Drawing for the job (mm, zero at the part's lowest x, y, z). A direction names the side the tool comes from. Round coordinates to 2 decimals unless told otherwise and drop trailing zeros. Order: outer loops, then holes, each group sorted by start corner. A loop starts at its lowest first (then second) coordinate and runs counter-clockwise, first axis right, second up. Notation, with made-up numbers: (45.25, -11) - (54.25, -11) arc R25 ccw to (54.25, 17) - close; hole circle Ø11 at (29, -39.75). An arc over 180 degrees is marked (long way). Put each result on its own line as item: value. Start each with the question number.
Item 1: Saw through at B-B on x = 20. List the corners of the cut face in (y, z).
Item 2: Saw through at C-C on z = 33.5. State how many separate pieces and enclosed holes the cut face has, plus the area to 3 significant figures.
Item 3: Probe probe 1 along X at (y, z) = (6.5, 29); probe 2 along Z at (x, y) = (6.5, 7); probe 3 along X at (y, z) = (1.2, 33). List the from-to ranges inside material, lowest first.
Item 4: Which spindle directions (+Z, -Z, +X, -X, +Y, -Y) get a long thin tool onto all of the face, cutting with end or side? Do the marked faces 1 and 2. Say none if no direction does.
Item 5: Mould opens along Z. For the marked faces 3, 4, 5 and 6 say: pulls with the +Z half, pulls with the -Z half, needs draft (parallel to the pull), parting line crosses it, or undercut.
Item 6: Saw through at A-A on y = 4.5. List the corners of the cut face in (x, z).
Item 7: Saw through at D-D on y = 6.75. List the corners of the cut face in (x, z), plus the area to 3 significant figures.
Item 8: Pin check, flat tips, straight feed: pin 1 Ø7 at (x, z) = (9, 33) entering from -Y; pin 2 Ø4 at (x, y) = (24.5, 1) entering from +Z; pin 3 Ø1.5 at (x, z) = (29, 32.5) entering from +Y; pin 4 Ø2 at (x, y) = (8, 2) entering from +Z. Stop position of each tip, or through.
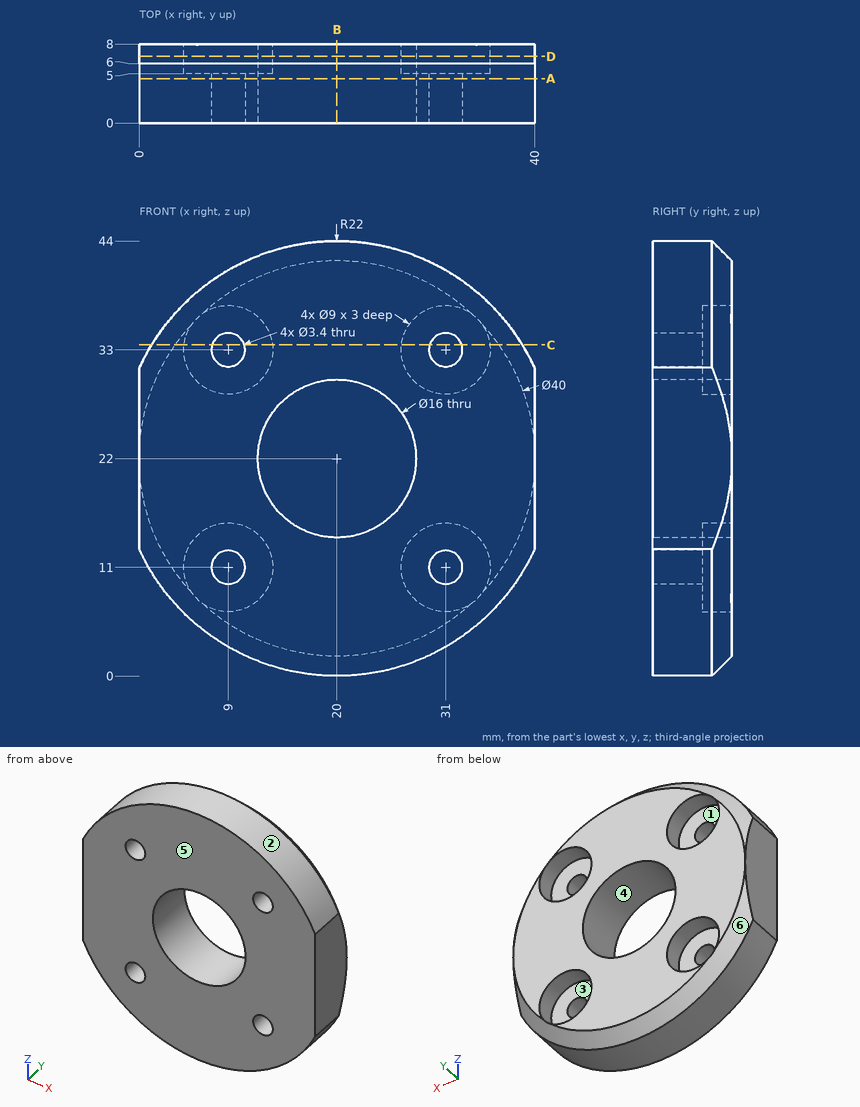
Results found:
1. outline: (0, 0) - (6, 0) - (8, 2) - (8, 14) - (0, 14) - close; (0, 30) - (8, 30) - (8, 42) - (6, 44) - (0, 44) - close
2. separate pieces: 3
2. enclosed holes: 0
2. area: 209 mm²
3. probe 1: x = 0 to 6.94, 11.06 to 16.13, 23.87 to 28.94, 33.06 to 40
3. probe 2: z = 5.91 to 7.26, 14.74 to 29.26, 36.74 to 38.09
3. probe 3: x = 0.95 to 7.3, 10.7 to 29.3, 32.7 to 39.05
4. face 1: +Y
4. face 2: +Z, +Y, -Y
5. face 3: undercut
5. face 4: undercut
5. face 5: needs draft
5. face 6: pulls with the -Z half
6. outline: (0, 12.83) arc R22 ccw to (40, 12.83) - (40, 31.17) arc R22 ccw to (0, 31.17) - close; hole circle Ø3.4 at (9, 11); hole circle Ø3.4 at (9, 33); hole circle Ø16 at (20, 22); hole circle Ø3.4 at (31, 11); hole circle Ø3.4 at (31, 33)
7. outline: (0, 14.82) arc R21.25 ccw to (40, 14.82) - (40, 29.18) arc R21.25 ccw to (0, 29.18) - close; hole circle Ø9 at (9, 11); hole circle Ø9 at (9, 33); hole circle Ø16 at (20, 22); hole circle Ø9 at (31, 11); hole circle Ø9 at (31, 33)
7. area: 939 mm²
8. pin 1: stops at y = 0
8. pin 2: stops at z = 43.86
8. pin 3: stops at y = 5
8. pin 4: stops at z = 41.05
